from build123d import *

# Parameters (mm, degrees)
F0_W      = 42
F0_H      = 19
F1_DEPTH  = 133
F2_DEPTH  = 25
F3_W      = 21
F3_H      = 42
F4_DEPTH  = 19
F5_R      = 9.5
F6_DEPTH  = 46.001
F7_W      = 21
F7_H      = 42
F8_DEPTH  = 19.001
F10_DEPTH = 3
F11_DEPTH = 19.001
F13_DEPTH = 22


with BuildPart() as f1:
    # F0 (on Right) → F1 (new body)
    with BuildSketch(Plane.YZ):
        with Locations((21, 9.5)):
            Rectangle(F0_W, F0_H)
    extrude(amount=F1_DEPTH)

    # F0 (on Right) → F2 (join)
    with BuildSketch(Plane.YZ):
        with BuildLine():
            Line((0, 41), (0, 19))
            Line((0, 19), (42, 19))
            Line((42, 19), (42, 41))
            ThreePointArc((42, 41), (21, 62), (0, 41))
        make_face()
    extrude(amount=F2_DEPTH)

    # F3 (on face) → F4 (join)
    with BuildSketch(Plane.XY.offset(19)):
        with Locations((-10.5, 21)):
            Rectangle(F3_W, F3_H)
    extrude(amount=-F4_DEPTH)

    # F5 (on face) → F6 (cut, through all)
    with BuildSketch(Plane.YZ.offset(25)):
        with Locations((21, 41)):
            Circle(F5_R)
    extrude(amount=-F6_DEPTH, mode=Mode.SUBTRACT)

    # F7 (on face) → F8 (cut, through all)
    with BuildSketch(Plane.XY.offset(19)):
        with Locations((122.5, 21)):
            Rectangle(F7_W, F7_H)
    extrude(amount=-F8_DEPTH, mode=Mode.SUBTRACT)

    # F9 (on face) → F10 (join)
    with BuildSketch(Plane.XY.offset(19)):
        with BuildLine():
            Line((87, 34), (43, 34))
            ThreePointArc((43, 34), (30, 21), (43, 8))
            Line((43, 8), (87, 8))
            ThreePointArc((87, 8), (100, 21), (87, 34))
        make_face()
        with BuildLine():
            ThreePointArc((43, 14.5), (36.5, 21), (43, 27.5))
            Line((43, 27.5), (87, 27.5))
            ThreePointArc((87, 27.5), (93.5, 21), (87, 14.5))
            Line((87, 14.5), (43, 14.5))
        make_face(mode=Mode.SUBTRACT)
    extrude(amount=F10_DEPTH)

    # F9 (on face) → F11 (cut, through all)
    with BuildSketch(Plane.XY.offset(19)):
        with BuildLine():
            Line((87, 27.5), (43, 27.5))
            ThreePointArc((43, 27.5), (36.5, 21), (43, 14.5))
            Line((43, 14.5), (87, 14.5))
            ThreePointArc((87, 14.5), (93.5, 21), (87, 27.5))
        make_face()
    extrude(amount=-F11_DEPTH, mode=Mode.SUBTRACT)

    # F12 (on face) → F13 (join)
    with BuildSketch(Plane(origin=(0, 42, 0), x_dir=(-1, 0, 0), z_dir=(0, 1, 0))):
        with BuildLine():
            Line((-100, 0), (21, 0))
            ThreePointArc((21, 0), (15.630878, 35.644074), (0, 68.124885))
            Line((0, 68.124885), (-100, 0))
        make_face()
    extrude(amount=F13_DEPTH)


solid = f1.part
Design review of the part built by this model. Coordinates are the model's own, in mm. A direction names the side the tool comes from. Give positions to 0.01 mm unless a question says otherwise; leave off trailing zeros. Order: outer loops, then holes, each group sorted by start corner. A loop starts at its lowest first (then second) coordinate and runs counter-clockwise, first axis right, second up. Notation, with made-up numbers: (42.25, 2) - (86.25, 2) arc R10 ccw to (86.25, 6) - close; hole circle Ø10 at (63, -18). An arc over 180 degrees is marked (long way). Write item = value, one per line. Start each with the question number.
Q1. Clearance check with flat-ended pins moving along their axes: pin 1 Ø21 at (x, y) = (50.5, 19.5) entering from +Z; pin 2 Ø1.5 at (x, z) = (72, 20) entering from -Y; pin 3 Ø24.5 at (y, z) = (21, 41) entering from +X. State where each tip first meets the part, or that it passes through.
Q2. Tool access review of faces 1 (the face through (-15.78, 52.85, 35.16)), 2 (the face through (46, 32, 0)), 3 (the face through (96, 42, 12)), 4 (the face through (0, 21, 31)), 5 (the face through (100, 21, 20)): name each direction out of +Z, -Z, +X, -X, +Y, -Y from which nothing blocks a thin tool from reaching the whole face with its end or side.
Q3. We need section B-B on z = 45. State the section outline as (x, y) points.
Q4. We need section C-C on x = 9. State the section outline as (y, z) points.
Q5. To check wall thickness, follow L1, parallel to Z at x = 7, y = 21; L2, parallel to Y at x = 73.5, z = 9; L3, parallel to Y at x = -6.5, z = 26.5. State the ranges of each line that lie inside material, in increasing order. Write a range as from..to.
Q6. We need section D-D on z = 59.5. State the section outline as (x, y) points, plus the area to 3 significant figures.
Q7. Mouldability with a two-part tool opening along X and no side actions: class faces 6 (the face through (65, 27.5, 11)), 7 (the face through (-21, 21, 10)), 8 (the face through (65, 8, 20)), 9 (the face through (93.5, 20.9, 11.2)) as released by +X, released by -X, zero draft, split by the parting line, or undercut.
Q8. We need section A-A on y = 21. State the section outline as (x, z) points.
Working result:
q1.pin_1 = 22
q1.pin_2 = 8
q1.pin_3 = 25
q2.face_1 = +Z, -X, +Y
q2.face_2 = -Z, +X, -X, +Y, -Y
q2.face_3 = +Z, +X, +Y
q2.face_4 = +Z, -X, -Y
q2.face_5 = +Z, +X
q3.outline = (-12.32, 42) - (33.94, 42) - (33.94, 64) - (-12.32, 64) - close; (0, 0.38) - (25, 0.38) - (25, 12.38) - (0, 12.38) - close; (0, 29.62) - (25, 29.62) - (25, 41.62) - (0, 41.62) - close
q4.outline = (0, 0) - (64, 0) - (64, 61.99) - (42, 61.99) - (42, 41) arc R21 ccw to (0, 41) - close; hole circle Ø19 at (21, 41)
q5.L1 = 0..31.5, 50.5..62
q5.L2 = 0..14.5, 27.5..64
q5.L3 = 42..64
q6.outline = (-5.36, 42) - (12.66, 42) - (12.66, 64) - (-5.36, 64) - close; (0, 11.06) - (25, 11.06) - (25, 30.94) - (0, 30.94) - close
q6.area = 893 mm²
q7.face_6 = undercut
q7.face_7 = released by -X
q7.face_8 = zero draft
q7.face_9 = undercut
q8.outline = (-21, 0) - (36.5, 0) - (36.5, 22) - (30, 22) - (30, 19) - (25, 19) - (25, 31.5) - (0, 31.5) - (0, 19) - (-21, 19) - close; (0, 50.5) - (25, 50.5) - (25, 62) - (0, 62) - close; (93.5, 0) - (112, 0) - (112, 19) - (100, 19) - (100, 22) - (93.5, 22) - close
